```python
from build123d import *

# Parameters (mm, degrees)
SKETCH1_W           = 75
SKETCH1_H           = 2
BOSS_EXTRUDE1_DEPTH = 10
SKETCH2_R           = 3.375
SKETCH2_R_2         = 1.375
BOSS_EXTRUDE2_DEPTH = 5
SKETCH3_R           = 1.375
CUT_EXTRUDE1_DEPTH  = 40.131189606


with BuildPart() as part:
    # Sketch1 → Boss-Extrude1 (new body)
    with BuildSketch(Plane.XY):
        with Locations((0, 1)):
            Rectangle(SKETCH1_W, SKETCH1_H)
    extrude(amount=BOSS_EXTRUDE1_DEPTH)

    # Sketch2 → Boss-Extrude2 (add)
    # profile 1 of 2: a face of its own
    with BuildSketch(Plane(origin=(0, 2, 0), x_dir=(1, 0, 0), z_dir=(0, 1, 0))):
        with Locations(Location((18.75, -5, 0), (0, 0, 90))):
            Circle(SKETCH2_R)
        with Locations(Location((18.75, -5, 0), (0, 0, 270))):
            Circle(SKETCH2_R_2, mode=Mode.SUBTRACT)
    # profile 2 of 2: a face of its own
    with BuildSketch(Plane(origin=(0, 2, 0), x_dir=(1, 0, 0), z_dir=(0, 1, 0))):
        with Locations(Location((-18.75, -5, 0), (0, 0, 90))):
            Circle(SKETCH2_R)
        with Locations(Location((-18.75, -5, 0), (0, 0, 90))):
            Circle(SKETCH2_R_2, mode=Mode.SUBTRACT)
    extrude(amount=BOSS_EXTRUDE2_DEPTH)

    # Sketch3 → Cut-Extrude1 (cut, through all)
    with BuildSketch(Plane(origin=(0, 2, 0), x_dir=(1, 0, 0), z_dir=(0, 1, 0))):
        with Locations(Location((18.75, -5, 0), (0, 0, 270))):
            Circle(SKETCH3_R)
        with Locations(Location((-18.75, -5, 0), (0, 0, 90))):
            Circle(SKETCH3_R)
    extrude(amount=-CUT_EXTRUDE1_DEPTH, mode=Mode.SUBTRACT)


solid = part.part
```
Part model, mm, in its own coordinate system. A direction names the side the tool comes from. Round coordinates to 2 decimals unless told otherwise and drop trailing zeros. Write each loop counter-clockwise with the first axis right and the second up, starting at its lowest first coordinate (ties: lowest second). Pieces come first, ordered by that corner, then holes. Notation, with made-up numbers: M 9.25,69.5 L 31.25,69.5 A16 ccw 31.25,76.5 Z; hole C -20,1.5 d5. An arc over 180 degrees is marked long. Answer as CSV lines item,"result". Start each with the question number.
1) Mould opens along X. For faces 3 (the face through (-19.76, 4.46, 1.78)), 4 (the face through (37.5, 1, 5)), 5 (the face through (20, 7, 4)) say: +X half, -X half, draft (parallel to the pull), parting line (faces both ways), or undercut.
2) Band-saw the part on A-A (z = 5). List the corners of the cut face in (x, y) (3 decimals), then the cut area to 3 significant figures.
3) Band-saw the part on D-D (x = -16). List the corners of the cut face in (y, z).
4) Drop flat-ended pins along their axis: pin 1 (1 mm diameter, centred on y = 5.5, z = 3, fed in from +X); pin 2 (3 mm diameter, centred on x = 10.5, z = 7.5, fed in from +Y); pin 3 (2 mm diameter, centred on y = 4.5, z = 2, fed in from -X). Give the stop position or say it passes through.
5) Which spindle directions (+Z, -Z, +X, -X, +Y, -Y) get a long thin tool onto all of the face, cutting with end or side? Do faces 1 (the face through (-17, 7, 5)), 2 (the face through (17.74, 4.46, 1.78)). Say none if no direction does.
6) Band-saw the part on B-B (y = 4). List the corners of the cut face in (x, z) (3 decimals).
7) Drill centre lines: L1, parallel to X at y = 4.55, z = 5 (3 decimals); L2, parallel to Z at x = -18.75, y = 5.6 (3 decimals); L3, parallel to Y at x = -5.5, z = 0.5. Where is each one in solid material? Low to high.
8) Band-saw the part on C-C (x = 18.75). List the corners of the cut face in (y, z) (3 decimals).
Worked out:
1,face 3,"undercut"
1,face 4,"+X half"
1,face 5,"draft"
2,outline,"M -37.5,0 L -20.125,0 L -20.125,7 L -22.125,7 L -22.125,2 L -37.5,2 Z; M -17.375,0 L 17.375,0 L 17.375,7 L 15.375,7 L 15.375,2 L -15.375,2 L -15.375,7 L -17.375,7 Z; M 20.125,0 L 37.5,0 L 37.5,2 L 22.125,2 L 22.125,7 L 20.125,7 Z"
2,area,"179 mm²"
3,outline,"M 0,0 L 2,0 L 2,3.04 L 7,3.04 L 7,6.96 L 2,6.96 L 2,10 L 0,10 Z"
4,pin 1,"x = 21.77"
4,pin 2,"y = 2"
4,pin 3,"x = -21.47"
5,face 1,"+Z, -Z, +X, -X, +Y"
5,face 2,"+Y"
6,outline,"C -18.75,5 d6.75; C 18.75,5 d6.75; hole C -18.75,5 d2.75; hole C 18.75,5 d2.75"
7,L1,"-22.125 to -20.125, -17.375 to -15.375, 15.375 to 17.375, 20.125 to 22.125"
7,L2,"1.625 to 3.625, 6.375 to 8.375"
7,L3,"0 to 2"
8,outline,"M 0,0 L 2,0 L 2,1.625 L 7,1.625 L 7,3.625 L 0,3.625 Z; M 0,6.375 L 7,6.375 L 7,8.375 L 2,8.375 L 2,10 L 0,10 Z"
